Autodesk Inventor part; units mm, degrees
ref_plane "YZ Plane" through (0, 0, 0) normal (1, 0, 0) x (0, 1, 0)
ref_plane "XY Plane" through (0, 0, 0) normal (0, 0, 1) x (1, 0, 0)
ref_plane "UCS1: YZ Plane" through (0, 0, 0) normal (1, 0, 0) x (0, 1, 0)
sketch "Sketch2" plane through (0, 0, 0) normal (1, 0, 0) x (0, 1, 0)
  circle A0 centre (0, -70) radius 26
  line L0 (25, -200) -> (-25, -200)
  line L1 (0, -70) -> (0, -200) construction
  line L2 (-25.9992, -70.2001) -> (-25, -200)
  line L3 (25.9992, -70.2001) -> (25, -200)
  circle A1 centre (0, 0) radius 25
  line L4 (-24.9974, 0.3571) -> (-25.9973, -69.6286)
  line L5 (24.9974, 0.3571) -> (25.9973, -69.6286)
  point P0 (25, 0)
  point P1 (-25, 0)
  dimension "d1" = 52
  dimension "d3" = 50
  dimension "d25" = 130
  dimension "d26" = 50
  dimension "d33" = 70
extrude "Extrusion1" add sketch "Sketch2" along normal blind 17.5 and the other way blind 27.5 contours A0
extrude "Extrusion2" add sketch "Sketch2" against normal blind 45 from surface at 17.5 contours L3 L0 L2 A0
sketch "Sketch5" plane through (17.5, -25, -200) normal (0, 0, -1) x (-1, 0, 0)
  circle A0 centre (22.5, 25) radius 10
  line L0 (45, 50) -> (45, 0)
  line L1 (45, 50) -> (0, 50)
  point P0 (17.5, 25)
  point P1 (45, 25)
  point P2 (-45, 0)
  point P3 (22.5, 50)
  dimension "d22" = 20
extrude "Extrusion4" cut sketch "Sketch5" against normal blind 60
ref_plane "Work Plane1" through (-5, 0, -70) normal (-1, 0, 0) x (0, 0, -1)
sketch "Sketch4" plane through (-5, 0, -70) normal (-1, 0, 0) x (0, 0, -1)
  circle A0 centre (-70, 0) radius 200
  line L0 (130, -25) -> (130, 25)
  line L1 (-270, 0) -> (130, 0)
  line L2 (130, 0) -> (130, 25)
  line L3 (130, 25) -> (0.2001, 25.9992)
  line L4 (130, 25) -> (130.19, 49.679)
  line L5 (130.19, 49.679) -> (123.719, 49.7288)
  point P0 (128.4298, 25.0121)
  point P1 (130, 0)
revolve "Revolution1" cut sketch "Sketch4" angle 360 about axis through (-5, 0, 200) along (0, 0, -1) contours L5 L4 L3 A0 | L3 L0 A0
extrude "Extrusion5" add sketch "Sketch2" along normal blind 17.5 and the other way blind 27.5 contours A0 L4 A1 L5
properties part number "shank_inventor"
For this review, take the finished solid that the model builds, in its own axes (mm). A direction names the side the tool comes from. Round coordinates to 2 decimals unless told otherwise and drop trailing zeros. Write each loop counter-clockwise with the first axis right and the second up, starting at its lowest first coordinate (ties: lowest second). Pieces come first, ordered by that corner, then holes. Notation, with made-up numbers: M 54,14.25 L 83,14.25 A12 ccw 83,31.25 Z; hole C 72.5,-2.5 d7. An arc over 180 degrees is marked long. Write item = value, one per line. Start each with the question number.
(1) For line 1 along X through (y, z) = (0, -176); line 2 along Y through (x, z) = (-5, -166.5); line 3 along Z through (x, y) = (3, 1.5), list the stretches that pass through material, from the lowest coordinate up.
(2) The part is to be moulded in two halves that separate along Y. For faces 3 (the face through (-27.5, 0, -98)), 4 (the face through (-5, 0, -140)), say which applies: +Y half, -Y half, draft (parallel to the pull), parting line (faces both ways), or undercut.
(3) We need section D-D (z = -29). Give the boundary of the cut face in (x, y), then the cut area to 3 significant figures.
(4) We need section C-C (x = -19.5). Give the boundary of the cut face in (y, z), then the cut area to 3 significant figures.
(5) For faces 1 (the face through (-14.54, 3, -170.29)), 2 (the face through (17.5, 0, -98)), list the 3-axis set-ups (+Z, -Z, +X, -X, +Y, -Y) from which the entire face can be reached by the end or side of a thin tool; tool diameter is ignored.
(6) We need section B-B (z = -155.5). Give the boundary of the cut face in (x, y), then the cut area to 3 significant figures.
(7) Clearance check with flat-ended pins moving along their axes: pin 1 Ø2 at (x, y) = (5.5, -11.5) entering from +Z; pin 2 Ø6 at (x, z) = (0, -27) entering from -Y; pin 3 Ø10 at (x, y) = (-4.5, -3.5) entering from -Z; pin 4 Ø10 at (x, y) = (-10, -9) entering from -Z. State where each tip first meets the part, or that it passes through.
(8) We need section A-A (y = 0). Give the boundary of the cut face in (x, z), then the cut area to 3 significant figures.
Results found:
q1.line_1 = -27.5 to -15, 5 to 17.5
q1.line_2 = -25.26 to -10, 10 to 25.26
q1.line_3 = -140 to -24.95
q2.face_3 = draft
q2.face_4 = undercut
q3.outline = M -27.5,-25.42 L 17.5,-25.42 L 17.5,25.42 L -27.5,25.42 Z
q3.area = 2,290 mm²
q4.outline = M -26,-70.2 L -25.02,-197.9 A199.47 ccw 25.02,-197.9 L 26,-70.2 A26 ccw 26,-69.63 L 25,0.31 A25 cw long -25,0.31 L -26,-69.63 A26 ccw Z
q4.area = 9,170 mm²
q5.face_1 = -Z
q5.face_2 = +Z, -Z, +X, +Y, -Y
q6.outline = M -27.5,-25.34 L 17.5,-25.34 L 17.5,25.34 L -27.5,25.34 Z; hole C -5,0 d20
q6.area = 1,970 mm²
q7.pin_1 = -21.65
q7.pin_2 = -25.43
q7.pin_3 = -140
q7.pin_4 = -199.75
q8.outline = M -27.5,-198.73 A200 ccw -15,-199.75 L -15,-140 L 5,-140 L 5,-199.75 A200 ccw 17.5,-198.73 L 17.5,-25 L -27.5,-25 Z
q8.area = 6,660 mm²
